The listing builds one solid part. Answer for the finished solid, in the listing's coordinates (mm). Face numbers are marked on the shaded views. A direction names the side the tool comes from. Round coordinates to 2 decimals unless told otherwise and drop trailing zeros. Loops run counter-clockwise (first coordinate to the right, second up) from the corner with the lowest first, then second, coordinate; pieces in that order, holes last. Notation, with made-up numbers: (10, -39) -> (50, -39) arc R27 cw to (50, 0) -> close; hole circle Ø9 at (59.5, -3). An arc over 180 degrees is marked (long way). Answer in a Markdown table with one row per item. Add a question column.
```python
from build123d import *

# Parameters (mm, degrees)
BOSS_EXTRUDE1_START     = 10
BOSS_EXTRUDE1_DEPTH     = 5
BOSS_EXTRUDE2_START     = -25
BOSS_EXTRUDE2_DEPTH     = 10
BOSS_EXTRUDE3_START     = 50
BOSS_EXTRUDE3_DEPTH     = 25
BOSS_EXTRUDE6_START     = -100
BOSS_EXTRUDE6_DEPTH     = 120
CUT_EXTRUDE1_DEPTH      = 243.699343574
CUT_EXTRUDE1_DEPTH_BACK = 243.699343574


with BuildPart() as part:
    # Sketch2 → Boss-Extrude1 (new body)
    with BuildSketch(Plane(origin=(0, 0, -40), x_dir=(-1, 0, 0), z_dir=(0, 0, -1)).offset(BOSS_EXTRUDE1_START)):
        Polygon((-55.5, 0), (-85.5, 0), (-85.5, -170), (39.5, -170), (39.5, 70), (-55.5, 70), align=None)
    extrude(amount=BOSS_EXTRUDE1_DEPTH)

    # Sketch3 → Boss-Extrude2 (add)
    with BuildSketch(Plane(origin=(0, 0, 0), x_dir=(0, 0, -1), z_dir=(1, 0, 0)).offset(BOSS_EXTRUDE2_START)):
        with BuildLine():
            Line((-56.504171272, 49.963866159), (-50.228142967, 26.541409655))
            ThreePointArc((-50.228142967, 26.541409655), (-41.254373695, 8.344405692), (-26, -5.033320997))
            Line((-26, -5.033320997), (50, -48.911941455))
            Line((50, -48.911941455), (55, -48.911941455))
            Line((55, -48.911941455), (55, -28.911941455))
            Line((55, -28.911941455), (50, -28.911941455))
            Line((50, -28.911941455), (50, 30))
            Line((50, 30), (55, 30))
            Line((55, 30), (55, 60))
            Line((55, 60), (42, 60))
            Line((42, 60), (42, 40))
            ThreePointArc((42, 40), (5.482100073, -1.640684178), (-40.568884704, 29.129600106))
            Line((-40.568884704, 29.129600106), (-46.844913009, 52.55205661))
            Line((-46.844913009, 52.55205661), (-56.504171272, 49.963866159))
        make_face()
    extrude(amount=-BOSS_EXTRUDE2_DEPTH)

    # Sketch3<3> → Boss-Extrude3 (add)
    with BuildSketch(Plane(origin=(0, 0, 0), x_dir=(0, 0, -1), z_dir=(1, 0, 0)).offset(BOSS_EXTRUDE3_START)):
        with BuildLine():
            Line((-56.504171272, 49.963866159), (-50.228142967, 26.541409655))
            ThreePointArc((-50.228142967, 26.541409655), (-41.254373695, 8.344405692), (-26, -5.033320997))
            Line((-26, -5.033320997), (50, -48.911941455))
            Line((50, -48.911941455), (55, -48.911941455))
            Line((55, -48.911941455), (55, -28.911941455))
            Line((55, -28.911941455), (50, -28.911941455))
            Line((50, -28.911941455), (50, 30))
            Line((50, 30), (55, 30))
            Line((55, 30), (55, 60))
            Line((55, 60), (42, 60))
            Line((42, 60), (42, 40))
            ThreePointArc((42, 40), (5.482100073, -1.640684178), (-40.568884704, 29.129600106))
            Line((-40.568884704, 29.129600106), (-46.844913009, 52.55205661))
            Line((-46.844913009, 52.55205661), (-56.504171272, 49.963866159))
        make_face()
    extrude(amount=-BOSS_EXTRUDE3_DEPTH)

    # Sketch4 → Boss-Extrude6 (add)
    with BuildSketch(Plane(origin=(0, 0, 0), x_dir=(1, 0, 0), z_dir=(0, 1, 0)).offset(BOSS_EXTRUDE6_START)):
        with BuildLine():
            Line((22.5, -15), (30, -15))
            Line((30, -15), (30, 50))
            Line((30, 50), (25, 50))
            Line((25, 50), (25, 55))
            Line((25, 55), (-25, 55))
            Line((-25, 55), (-25, 50))
            Line((-25, 50), (-30, 50))
            Line((-30, 50), (-30, -15))
            Line((-30, -15), (-22.5, -15))
            Line((-22.5, -15), (-22.5, 0))
            ThreePointArc((-22.5, 0), (0, 22.5), (22.5, 0))
            Line((22.5, 0), (22.5, -15))
        make_face()
    extrude(amount=-BOSS_EXTRUDE6_DEPTH)

    # Sketch3<8> → Cut-Extrude1 (cut, two sides: drawn at the far end of the back side and taken through both)
    with BuildSketch(Plane(origin=(0, 0, 0), x_dir=(0, 0, -1), z_dir=(1, 0, 0)).offset(-CUT_EXTRUDE1_DEPTH_BACK)):
        Polygon((15, -100), (50, -100), (50, -80), (-50, -80), (-50, -245), (50, -245), (50, -150), (45, -150), (30, -175.980762114), (30, -220), (-3.452994616, -220), (-15, -200), (-15, -151.961524227), align=None)
    extrude(amount=CUT_EXTRUDE1_DEPTH + CUT_EXTRUDE1_DEPTH_BACK, mode=Mode.SUBTRACT)


solid = part.part
```
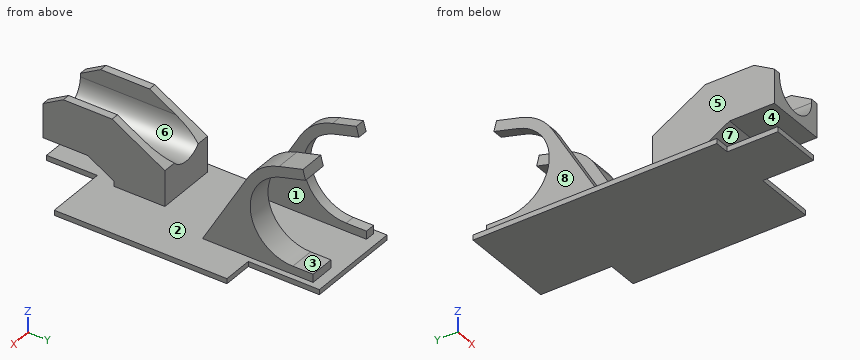
Item 1: Flat-ended cylindrical pins translate along their axes: P1, Ø6, axis at x = 27, y = -176, coming from the +Z side; P2, Ø5.5, axis at x = 57, z = -51.5, coming from the -Y side; P3, Ø2.5, axis at y = -188, z = -51.5, coming from the +X side. Find the tip coordinate at first contact, or state that the pin passes through.
Item 2: Section B-B, the plane x = 0 is taken. Write down the section's boundary in (y, z), and give its area (3 significant figures).
Item 3: Consider L1, parallel to X at y = -18, z = -24.5; L2, parallel to Z at x = 79, y = -108.5; L3, parallel to X at y = -182, z = 6. Determine where each line is inside the solid, lowest interval first. Write a range as from..to.
Item 4: Section D-D, the plane y = -132 is taken. Write down the section's boundary in (x, z).
Item 5: The mould has two halves that part along X. Classify the marked faces 6, 7 and 8: +X half, -X half, draft (parallel to the pull), parting line (faces both ways), or undercut.
Item 6: Section C-C, the plane z = 37 is taken. Write down the section's boundary in (x, y).
Item 7: Section A-A, the plane z = -11 is taken. Write down the section's boundary in (x, y), and give its area (3 significant figures).
Item 8: For the marked faces 1, 2, 3, 4 and 5, determine the directions among +Z, -Z, +X, -X, +Y, -Y from which every point of the face is accessible in a straight line to the end or side of a thin tool.
Here are the results:
| question | item | result |
|---|---|---|
| 1 | P1 | stops at z = 15 |
| 1 | P2 | stops at y = -170 |
| 1 | P3 | stops at x = 25 |
| 2 | outline | (-220, -55) -> (70, -55) -> (70, -50) -> (-100, -50) -> (-100, -22.5) -> (-220, -22.5) -> (-220, -30) -> (-175.98, -30) -> (-150, -45) -> (-150, -50) -> (-220, -50) -> close |
| 2 | area | 3,540 mm² |
| 3 | L1 | x = -35..-25, 25..50 |
| 3 | L2 | z = -55..-50 |
| 3 | L3 | x = -30..-22.5, 22.5..30 |
| 4 | outline | (-39.5, -55) -> (85.5, -55) -> (85.5, -50) -> (30, -50) -> (30, 3.48) -> (22.5, 3.48) -> (22.5, 0) arc R22.5 cw to (-22.5, 0) -> (-22.5, 3.48) -> (-30, 3.48) -> (-30, -50) -> (-39.5, -50) -> close |
| 5 | face 6 | undercut |
| 5 | face 7 | draft |
| 5 | face 8 | -X half |
| 6 | outline | (-35, 3.46) -> (-25, 3.46) -> (-25, 20.13) -> (-35, 20.13) -> close; (25, 3.46) -> (50, 3.46) -> (50, 20.13) -> (25, 20.13) -> close |
| 7 | outline | (-35, -26.4) -> (-25, -26.4) -> (-25, -0.53) -> (-35, -0.53) -> close; (-30, -220) -> (-19.63, -220) -> (-19.63, -106.93) -> (-30, -106.93) -> close; (19.63, -220) -> (30, -220) -> (30, -106.93) -> (19.63, -106.93) -> close; (25, -26.4) -> (50, -26.4) -> (50, -0.53) -> (25, -0.53) -> close |
| 7 | area | 3,250 mm² |
| 8 | face 1 | +Z, +Y |
| 8 | face 2 | none |
| 8 | face 3 | +X, -X, +Y |
| 8 | face 4 | +X, -X, -Y |
| 8 | face 5 | +Z, -X, -Y |
